from build123d import *

# Parameters (mm, degrees)
SKETCH012_W                   = 88
SKETCH012_H                   = 48
PAD005_DEPTH                  = 4
SKETCH013_W                   = 81
SKETCH013_H                   = 41
PAD006_DEPTH                  = 2
POCKET007_DEPTH               = 2
POCKET007_MIRRORED009_2_DEPTH = 2
POCKET008_DEPTH               = 2
SKETCH016_R                   = 1.6
POCKET009_DEPTH               = 206.8392433701
SKETCH016_MIRRORED011_2_R     = 1.6
POCKET009_MIRRORED011_2_DEPTH = 206.8392433701
SKETCH017_R                   = 4
POCKET010_DEPTH               = 3
SKETCH017_MIRRORED013_2_R     = 4
POCKET010_MIRRORED013_2_DEPTH = 3
SKETCH018_W                   = 100.342552
SKETCH018_H                   = 57.696968
POCKET011_DEPTH               = 1
POCKET012_DEPTH               = 205.7296725906
POCKET012_MIRRORED015_2_DEPTH = 205.7296725906
POCKET008_MIRRORED017_2_DEPTH = 2


with BuildPart() as part:
    # Sketch012 → Pad005 (new body)
    with BuildSketch(Plane.XY):
        Rectangle(SKETCH012_W, SKETCH012_H)
    extrude(amount=PAD005_DEPTH)

    # Sketch013 (on Face6 of Pad005) → Pad006 (join)
    with BuildSketch(Plane.XY.offset(4)):
        Rectangle(SKETCH013_W, SKETCH013_H)
    extrude(amount=PAD006_DEPTH)

    # Sketch014 (on Face11 of Pad006) → Pocket007 (cut)
    with BuildSketch(Plane.XY.offset(6)):
        Polygon((0, 0), (-40.5, 0), (-40.5, 11.9644660941), (-35.5, 11.9644660941), (-31.964466094, 15.5), (-31.964466094, 20.5), (0, 20.5), align=None)
    pocket007 = extrude(amount=-POCKET007_DEPTH, mode=Mode.SUBTRACT)

    # Sketch014 Mirrored009 2 → Pocket007 Mirrored009 2 (cut)
    with BuildSketch(Plane(origin=(0, 0, 6), x_dir=(-1, 0, 0), z_dir=(0, 0, -1))):
        Polygon((0, 0), (-40.5, 0), (-40.5, 11.9644660941), (-35.5, 11.9644660941), (-31.964466094, 15.5), (-31.964466094, 20.5), (0, 20.5), align=None)
    pocket007_mirrored009_2 = extrude(amount=POCKET007_MIRRORED009_2_DEPTH, mode=Mode.SUBTRACT)

    # Mirrored010: Pocket007, Pocket007 Mirrored009 2 across Sketch014 H_Axis
    add(pocket007.mirror(Plane(origin=(0, 0, 6), x_dir=(0, 0, 1), z_dir=(0, 1, 0))), mode=Mode.SUBTRACT)
    add(pocket007_mirrored009_2.mirror(Plane(origin=(0, 0, 6), x_dir=(0, 0, 1), z_dir=(0, 1, 0))), mode=Mode.SUBTRACT)

    # Sketch015 (on Face20 of MultiTransform004) → Pocket008 (cut)
    with BuildSketch(Plane.XY.offset(6)):
        Polygon((-40.5, 17.5), (-40.5, 20.5), (-37.5, 20.5), align=None)
    pocket008 = extrude(amount=-POCKET008_DEPTH, mode=Mode.SUBTRACT)

    # Sketch016 (on Face4 of Pocket008) → Pocket009 (cut, through all)
    with BuildSketch(Plane(origin=(0, 0, 0), x_dir=(1, 0, 0), z_dir=(0, 0, -1))):
        with Locations((-35.75, 15.75)):
            Circle(SKETCH016_R)
    pocket009 = extrude(amount=-POCKET009_DEPTH, mode=Mode.SUBTRACT)

    # Sketch016 Mirrored011 2 → Pocket009 Mirrored011 2 (cut, through all)
    with BuildSketch(Plane(origin=(0, 0, 0), x_dir=(-1, 0, 0), z_dir=(0, 0, 1))):
        with Locations((-35.75, 15.75)):
            Circle(SKETCH016_MIRRORED011_2_R)
    pocket009_mirrored011_2 = extrude(amount=POCKET009_MIRRORED011_2_DEPTH, mode=Mode.SUBTRACT)

    # Mirrored012: Pocket009, Pocket009 Mirrored011 2 across Sketch016 H_Axis
    add(pocket009.mirror(Plane(origin=(0, 0, 0), x_dir=(0, 0, -1), z_dir=(0, -1, 0))), mode=Mode.SUBTRACT)
    add(pocket009_mirrored011_2.mirror(Plane(origin=(0, 0, 0), x_dir=(0, 0, -1), z_dir=(0, -1, 0))), mode=Mode.SUBTRACT)

    # Sketch017 (on Face4 of MultiTransform005) → Pocket010 (cut)
    with BuildSketch(Plane(origin=(0, 0, 0), x_dir=(1, 0, 0), z_dir=(0, 0, -1))):
        with Locations((-35.75, 15.75)):
            Circle(SKETCH017_R)
    pocket010 = extrude(amount=-POCKET010_DEPTH, mode=Mode.SUBTRACT)

    # Sketch017 Mirrored013 2 → Pocket010 Mirrored013 2 (cut)
    with BuildSketch(Plane(origin=(0, 0, 0), x_dir=(-1, 0, 0), z_dir=(0, 0, 1))):
        with Locations((-35.75, 15.75)):
            Circle(SKETCH017_MIRRORED013_2_R)
    pocket010_mirrored013_2 = extrude(amount=POCKET010_MIRRORED013_2_DEPTH, mode=Mode.SUBTRACT)

    # Mirrored014: Pocket010, Pocket010 Mirrored013 2 across Sketch017 H_Axis
    add(pocket010.mirror(Plane(origin=(0, 0, 0), x_dir=(0, 0, -1), z_dir=(0, -1, 0))), mode=Mode.SUBTRACT)
    add(pocket010_mirrored013_2.mirror(Plane(origin=(0, 0, 0), x_dir=(0, 0, -1), z_dir=(0, -1, 0))), mode=Mode.SUBTRACT)

    # Sketch018 (on Face4 of MultiTransform006) → Pocket011 (cut)
    with BuildSketch(Plane(origin=(0, 0, 0), x_dir=(1, 0, 0), z_dir=(0, 0, -1))):
        with Locations((-0.467655, 0.399981)):
            Rectangle(SKETCH018_W, SKETCH018_H)
    extrude(amount=-POCKET011_DEPTH, mode=Mode.SUBTRACT)

    # Sketch019 (on Face2 of Pocket011) → Pocket012 (cut, through all)
    with BuildSketch(Plane(origin=(0, 0, 1), x_dir=(1, 0, 0), z_dir=(0, 0, -1))):
        Polygon((-44, 18), (-38, 24), (-44, 24), align=None)
    pocket012 = extrude(amount=-POCKET012_DEPTH, mode=Mode.SUBTRACT)

    # Sketch019 Mirrored015 2 → Pocket012 Mirrored015 2 (cut, through all)
    with BuildSketch(Plane(origin=(0, 0, 1), x_dir=(-1, 0, 0), z_dir=(0, 0, 1))):
        Polygon((-44, 18), (-38, 24), (-44, 24), align=None)
    pocket012_mirrored015_2 = extrude(amount=POCKET012_MIRRORED015_2_DEPTH, mode=Mode.SUBTRACT)

    # Mirrored016: Pocket012, Pocket012 Mirrored015 2 across Sketch019 H_Axis
    add(pocket012.mirror(Plane(origin=(0, 0, 1), x_dir=(0, 0, -1), z_dir=(0, -1, 0))), mode=Mode.SUBTRACT)
    add(pocket012_mirrored015_2.mirror(Plane(origin=(0, 0, 1), x_dir=(0, 0, -1), z_dir=(0, -1, 0))), mode=Mode.SUBTRACT)

    # Sketch015 Mirrored017 2 → Pocket008 Mirrored017 2 (cut)
    with BuildSketch(Plane(origin=(0, 0, 6), x_dir=(-1, 0, 0), z_dir=(0, 0, -1))):
        Polygon((-40.5, 17.5), (-40.5, 20.5), (-37.5, 20.5), align=None)
    pocket008_mirrored017_2 = extrude(amount=POCKET008_MIRRORED017_2_DEPTH, mode=Mode.SUBTRACT)

    # Mirrored018: Pocket008, Pocket008 Mirrored017 2 across Sketch015 H_Axis
    add(pocket008.mirror(Plane(origin=(0, 0, 6), x_dir=(0, 0, 1), z_dir=(0, 1, 0))), mode=Mode.SUBTRACT)
    add(pocket008_mirrored017_2.mirror(Plane(origin=(0, 0, 6), x_dir=(0, 0, 1), z_dir=(0, 1, 0))), mode=Mode.SUBTRACT)


with BuildPart() as part_1:
    # Body001 placement: moved
    add(part.part.moved(Location((0, 0, -2.6))))


solid = part_1.part
CAD build for the part. Positions are in the model's coordinates, mm. A direction names the side the tool comes from. Round coordinates to 2 decimals unless told otherwise and drop trailing zeros. Order: outer loops, then holes, each group sorted by start corner. A loop starts at its lowest first (then second) coordinate and runs counter-clockwise, first axis right, second up. Notation, with made-up numbers: (31, 15) - (63, 15) arc R9 ccw to (63, 26) - close; hole circle Ø1 at (38.5, 68). An arc over 180 degrees is marked (long way). Return JSON: item names as keys, results as strings.
(1) Cut at A-A (z = 2.4). Give the cut face in (x, y).
Answer key:
{"outline": "(-40.5, -17.5) - (-37.5, -20.5) - (-31.96, -20.5) - (-31.96, -15.5) - (-35.5, -11.96) - (-40.5, -11.96) - close; (-40.5, 11.96) - (-35.5, 11.96) - (-31.96, 15.5) - (-31.96, 20.5) - (-37.5, 20.5) - (-40.5, 17.5) - close; (31.96, -20.5) - (37.5, -20.5) - (40.5, -17.5) - (40.5, -11.96) - (35.5, -11.96) - (31.96, -15.5) - close; (31.96, 15.5) - (35.5, 11.96) - (40.5, 11.96) - (40.5, 17.5) - (37.5, 20.5) - (31.96, 20.5) - close; hole circle Ø3.2 at (-35.75, -15.75); hole circle Ø3.2 at (-35.75, 15.75); hole circle Ø3.2 at (35.75, -15.75); hole circle Ø3.2 at (35.75, 15.75)"}
(2) Cut at C-C (x = -19). Give the cut face in (y, z), then the cut area to 3 significant figures.
Answer key:
{"outline": "(-24, -1.6) - (24, -1.6) - (24, 1.4) - (-24, 1.4) - close", "area": "144 mm^2"}
(3) Pin check, flat tips, straight feed: pin 1 Ø4 at (x, y) = (-12, 2.5) entering from +Z; pin 2 Ø1 at (x, z) = (-34.5, 2.5) entering from +Y; pin 3 Ø2 at (y, z) = (-17, 2.5) entering from +X; pin 4 Ø3 at (x, y) = (35.75, 15.75) entering from +Z. Stop position of each tip, or through.
Answer key:
{"pin 1": "stops at z = 1.4", "pin 2": "stops at y = 20.5", "pin 3": "stops at x = 40.5", "pin 4": "passes through"}
(4) Cut at B-B (y = -5). Give the cut face in (x, z), then the cut area to 3 significant figures.
Answer key:
{"outline": "(-44, -1.6) - (44, -1.6) - (44, 1.4) - (-44, 1.4) - close", "area": "264 mm^2"}
(5) Tool access for faces 1 (the face through (-38, -11.964, 2)), 2 (the face through (-39, -19, 2)), 3 (the face through (35, 20.5, 2)), 4 (the face through (38.7, 18.45, -0.61)), 5 (the face through (40.5, -15, 2)): list every direction of +Z, -Z, +X, -X, +Y, -Y with a clear straight run to the whole face (end or side of a thin tool).
Answer key:
{"face 1": "+Z, +X, -X", "face 2": "+Z, -X, -Y", "face 3": "+Z, +X, -X, +Y", "face 4": "-Z", "face 5": "+Z, +X, +Y, -Y"}
(6) Wall check: probe 1 along Y at (x, z) = (-35.75, 2.75); probe 2 along X at (y, z) = (-15.75, -0.5); probe 3 along Y at (x, z) = (-33.5, -0.35). Give the ranges that are in metal, low to high. Write a range as from..to.
Answer key:
{"probe 1": "y = -20.5..-17.35, -14.15..-11.96, 11.96..14.15, 17.35..20.5", "probe 2": "x = -44..-39.75, -31.75..31.75, 39.75..44", "probe 3": "y = -24..-19.06, -12.44..12.44, 19.06..24"}
